from build123d import *

# Parameters (mm, degrees)
F1_DEPTH    = 241.3
F2_W        = 254
F2_H        = 190.5
F3_DEPTH    = 25.4
F5_DEPTH    = 508
F6_T1_DEPTH = 78.0207478943
F7_T1_DEPTH = 78.0207478943


# Not quite as in the source:
# - a fillet or chamfer that OpenCascade refuses, or shapes differently, is made with other operations: its cross-section is extruded or revolved along the edge and cut away or added


with BuildPart() as f1:
    # F0 (on Top) → F1 (new body)
    with BuildSketch(Plane.XY):
        Polygon((0, 12.7), (0, 0), (76.2, 0), (76.2, 25.4), (-76.2, 289.3645430735), (-87.1985226281, 283.0145430735), (63.5, 21.9970452561), (63.5, 12.7), align=None)
    extrude(amount=F1_DEPTH)

    # F2 (on face) → F3 (cut)
    with BuildSketch(Plane(origin=(68.1485226281, 39.3455678842, 0), x_dir=(-0.5, 0.8660254038, 0), z_dir=(0.8660254038, 0.5, 0))):
        with Locations((136.2970452561, 120.65)):
            Rectangle(F2_W, F2_H)
    extrude(amount=-F3_DEPTH, mode=Mode.SUBTRACT)

    # F4 (on face) → F5 (cut)
    with BuildSketch(Plane.XY.offset(241.3)):
        Polygon((-81.9939685629, 281.6199870148), (65.9347099118, 25.4), (71.8005932508, 25.4), (-77.5945560587, 284.1599890084), align=None)
    extrude(amount=-F5_DEPTH, mode=Mode.SUBTRACT)

    # F6: chamfer of 12.7 on 1 edges, made by hand

    # F6_s2 → F6_t1 (cut)
    with BuildSketch(Plane(origin=(96.4332361634, 55.6757548578, 0), x_dir=(0, 0, 1), z_dir=(-0.8660254038, -0.5, 0))):
        Polygon((0, 275.9970452561), (12.7, 288.6970452561), (0, 288.6970452561), align=None)
    extrude(amount=F6_T1_DEPTH, mode=Mode.SUBTRACT)

    # F7: chamfer of 12.7 on 1 edges, made by hand

    # F7_s2 → F7_t1 (cut)
    with BuildSketch(Plane(origin=(96.4332361634, 55.6757548578, 0), x_dir=(0, 0, 1), z_dir=(-0.8660254038, -0.5, 0))):
        Polygon((241.3, 275.9970452561), (228.6, 288.6970452561), (241.3, 288.6970452561), align=None)
    extrude(amount=F7_T1_DEPTH, mode=Mode.SUBTRACT)


solid = f1.part
Check sheet for the modelled part. Datum: model origin and axes. Units: mm. A direction names the side the tool comes from. Give positions to 0.01 mm unless a question says otherwise; leave off trailing zeros. Order: outer loops, then holes, each group sorted by start corner. A loop starts at its lowest first (then second) coordinate and runs counter-clockwise, first axis right, second up. Notation, with made-up numbers: (48, 32) - (106, 32) arc R9 cw to (106, 44) - close; hole circle Ø1 at (86.5, 4.25). An arc over 180 degrees is marked (long way). Answer as CSV lines item,"result".
1. Section check C-C (y = 120.5). Record the boundary of the cut face in (x, z), then the cut area to 3 significant figures.
Result sheet:
outline,"(6.63, 0) - (11.03, 0) - (11.03, 25.4) - (6.63, 25.4) - close; (6.63, 215.9) - (11.03, 215.9) - (11.03, 241.3) - (6.63, 241.3) - close; (16.89, 0) - (21.29, 0) - (21.29, 25.4) - (16.89, 25.4) - close; (16.89, 215.9) - (21.29, 215.9) - (21.29, 241.3) - (16.89, 241.3) - close"
area,"447 mm²"
2. Section check A-A (z = 80). Record the boundary of the cut face in (x, y).
Result sheet:
outline,"(-87.2, 283.01) - (-74.5, 261.02) - (-71.2, 262.92) - (-81.99, 281.62) - (-77.59, 284.16) - (-66.8, 265.46) - (-63.5, 267.37) - (-76.2, 289.36) - close; (0, 0) - (76.2, 0) - (76.2, 25.4) - (63.5, 47.4) - (60.2, 45.49) - (71.8, 25.4) - (65.93, 25.4) - (55.8, 42.95) - (52.5, 41.05) - (63.5, 22) - (63.5, 12.7) - (0, 12.7) - close"
3. Go/stop test with flat-tipped pins: P1, Ø4.5, axis at x = 68.5, z = 120, coming from the +Y side; P2, Ø4, axis at y = 7, z = 134.5, coming from the -X side; P3, Ø10, axis at x = 30, z = 200, coming from the +Y side; P4, Ø10, axis at x = -34, z = 208, coming from the +Y side. Record where each tip stops, or that it passes through.
Result sheet:
P1,"y = 42.63"
P2,"x = 0"
P3,"y = 12.7"
P4,"through"
4. Section check D-D (z = 225). Record the boundary of the cut face in (x, y), then the cut area to 3 significant figures.
Result sheet:
outline,"(-87.2, 283.01) - (63.5, 22) - (63.5, 12.7) - (0, 12.7) - (0, 0) - (76.2, 0) - (76.2, 25.4) - (-76.2, 289.36) - close; hole (-81.99, 281.62) - (65.93, 25.4) - (71.8, 25.4) - (-77.59, 284.16) - close"
area,"3,450 mm²"
5. Tool access check on faces 4 (the face through (-1.85, 152.97, 229.58)), 5 (the face through (76.2, 13, 119)), 6 (the face through (32, 12.7, 119)). Record the directions out of +Z, -Z, +X, -X, +Y, -Y that give a thin tool (end or side, any length) a straight path to the whole face; none if there is none.
Result sheet:
face 4,"+Z, -Z"
face 5,"+Z, -Z, +X, +Y, -Y"
face 6,"+Z, -Z, -X"
6. Mould release check, pull along Z, two halves, no side actions. Record for faces 1 (the face through (0, 6, 119)), 2 (the face through (-80.847, 279.247, 235.039)), 3 (the face through (-8, 150, 215.9)): released by +Z, released by -Z, zero draft, split by the parting line, or undercut.
Result sheet:
face 1,"zero draft"
face 2,"released by +Z"
face 3,"undercut"
7. Scan lines: probe 1 along Y at (x, z) = (50.5, 190); probe 2 along Z at (x, y) = (-2, 137); probe 3 along X at (y, z) = (245.5, 17). Record each from-to range of solid material in increasing order. Write a range as from..to.
Result sheet:
probe 1,"0..12.7"
probe 2,"0..25.4, 215.9..241.3"
probe 3,"-65.54..-61.14, -55.27..-50.87"
8. Section check B-B (x = -25.5). Record the boundary of the cut face in (y, z).
Result sheet:
outline,"(176.15, 0) - (183.77, 0) - (183.77, 25.4) - (176.15, 25.4) - close; (176.15, 215.9) - (183.77, 215.9) - (183.77, 241.3) - (176.15, 241.3) - close; (193.93, 0) - (201.55, 0) - (201.55, 25.4) - (193.93, 25.4) - close; (193.93, 215.9) - (201.55, 215.9) - (201.55, 241.3) - (193.93, 241.3) - close"
